Geometry: final body of the model. Coordinates: model frame, mm. A direction names the side the tool comes from. Coordinates: 2 decimals unless noted, no trailing zeros. Write each loop counter-clockwise with the first axis right and the second up, starting at its lowest first coordinate (ties: lowest second). Pieces come first, ordered by that corner, then holes. Notation, with made-up numbers: (-2.5, 22.5) - (48.5, 22.5) arc R10 cw to (48.5, 27.5) - close; hole circle Ø5 at (81, 62). An arc over 180 degrees is marked (long way). Answer as a JSON object with one key per item and string values. Group by question number.
Item 1: Set-up query: faces 1 (the flat face through (-9.5, 19, 3)), 2 (the flat face through (0, 5.65, 13)), 3 (the flat face through (7.825, 19, 16)). Return all of +Z, -Z, +X, -X, +Y, -Y with unobstructed straight access to the full face (end or side cutting, diameter ignored); none if empty.
Item 2: First-contact query: pin 1 Ø1.1 at (x, z) = (13, 3.5) entering from +Y; pin 2 Ø8 at (x, y) = (-20.5, 6.5) entering from +Z; pin 3 Ø3.5 at (x, y) = (20.5, 15.5) entering from -Z. Flat tips, straight axial feed; report the tip coordinate or a pass-through.
Item 3: Section C-C on z = -17.3. Return loops of the section in (x, y) (3 decimals), and give its area (3 significant figures).
Item 4: Line query: line 1 along X through (y, z) = (17.5, 3) (3 decimals); line 2 along Z through (x, y) = (2.5, 11); line 3 along X through (y, z) = (8.5, 0.5) (3 decimals). Output: solid intervals per line, ascending. Write a range as from..to.
Item 5: Section A-A on y = 10. Return loops of the section in (x, z) (3 decimals), and give its area (3 significant figures).
Item 6: Mould query, pull axis Z, two halves, no side actions, for faces 4 (the flat face through (0, 13.65, -17)), 5 (the flat face through (-0.1, 17.7, 18.85)), 6 (the flat face through (7.825, 13, -16)), 7 (the cylindrical face through (-0.06, 6.51, 9.75)). Classes: pulls with the +Z half, pulls with the -Z half, needs draft (parallel to the pull), parting line crosses it, or undercut.
Item 7: Section B-B on x = 0. Return loops of the section in (y, z), and give its area (3 significant figures).
```python
from build123d import *

# Parameters (mm, degrees)
SKETCH1_W             = 60
SKETCH1_H             = 18
BOSS_EXTRUDE1_DEPTH   = 26
SKETCH2_R             = 3.85
EYESHAFT_HOLES_DEPTH  = 15
EYESHAFT_FILLET_R     = 3
SKETCH5_W             = 5
SKETCH5_H             = 2.2
FRONT_LEG_HOLES_DEPTH = 13
SKETCH7_W             = 10.2
SKETCH7_H             = 3.3
BACK_LEGS_DEPTH       = 13
SKETCH18_W            = 15.65
SKETCH18_H            = 35.9
SERVO_BLOCK_DEPTH     = 26
SKETCH19_W            = 11.75
SKETCH19_H            = 32.2
SERVO_ARMS_DEPTH      = 9.35
SKETCH20_W            = 11.75
SKETCH20_H            = 23.9
CUT_EXTRUDE10_DEPTH   = 15
FILLET4_R             = 5
CHAMFER1_SIZE         = 1
SKETCH21_W            = 9
SKETCH21_H            = 4
CUT_EXTRUDE11_DEPTH   = 15
FILLET5_R             = 3
SKETCH22_R            = 0.75
CUT_EXTRUDE12_DEPTH   = 3
FILLET6_R             = 5
SKETCH23_W            = 15.65
SKETCH23_H            = 10
BOSS_EXTRUDE3_DEPTH   = 4
DOVE_TAIL_DEPTH       = 8
FILLET8_R             = 3.8
FILLET9_R             = 2


with BuildPart() as part:
    # Sketch1 → Boss-Extrude1 (new body)
    with BuildSketch(Plane(origin=(0, 0, 0), x_dir=(1, 0, 0), z_dir=(0, 1, 0))):
        Rectangle(SKETCH1_W, SKETCH1_H)
    extrude(amount=BOSS_EXTRUDE1_DEPTH)

    # Sketch2 → Eyeshaft holes (cut)
    with BuildSketch(Plane(origin=(0, 26, 0), x_dir=(1, 0, 0), z_dir=(0, 1, 0))):
        with Locations(Location((-22, -3, 0), (0, 0, 270))):
            Circle(SKETCH2_R)
        with Locations(Location((22, -3, 0), (0, 0, 270))):
            Circle(SKETCH2_R)
    extrude(amount=-EYESHAFT_HOLES_DEPTH, mode=Mode.SUBTRACT)

    # Eyeshaft Fillet
    eyeshaft_fillet_edges = [part.edges().sort_by_distance(p)[0] for p in [
        (-22, 11, -0.85),
        (22, 11, -0.85),
    ]]
    fillet(eyeshaft_fillet_edges, radius=EYESHAFT_FILLET_R)

    # Sketch5 → Front leg holes (cut)
    with BuildSketch(Plane(origin=(0, 26, 0), x_dir=(1, 0, 0), z_dir=(0, 1, 0))):
        with Locations((-12, -3)):
            Rectangle(SKETCH5_W, SKETCH5_H)
        with Locations((12, -3)):
            Rectangle(SKETCH5_W, SKETCH5_H)
    extrude(amount=-FRONT_LEG_HOLES_DEPTH, mode=Mode.SUBTRACT)

    # Sketch7 → Back Legs (cut)
    with BuildSketch(Plane(origin=(0, 26, 0), x_dir=(1, 0, 0), z_dir=(0, 1, 0))):
        with Locations((-13.9, 5.4)):
            Rectangle(SKETCH7_W, SKETCH7_H)
        with Locations((13.9, 5.4)):
            Rectangle(SKETCH7_W, SKETCH7_H)
    extrude(amount=-BACK_LEGS_DEPTH, mode=Mode.SUBTRACT)

    # Sketch18 → Servo Block (add)
    with BuildSketch(Plane(origin=(0, 26, 0), x_dir=(1, 0, 0), z_dir=(0, 1, 0))):
        with Locations((0, 3.1)):
            Rectangle(SKETCH18_W, SKETCH18_H)
    extrude(amount=-SERVO_BLOCK_DEPTH)

    # Sketch19 → Servo Arms (cut)
    with BuildSketch(Plane(origin=(0, 26, 0), x_dir=(1, 0, 0), z_dir=(0, 1, 0))):
        with Locations((0, 3.1)):
            Rectangle(SKETCH19_W, SKETCH19_H)
    extrude(amount=-SERVO_ARMS_DEPTH, mode=Mode.SUBTRACT)

    # Sketch20 → Cut-Extrude10 (cut)
    with BuildSketch(Plane(origin=(0, 16.65, 0), x_dir=(1, 0, 0), z_dir=(0, 1, 0))):
        with Locations((0, 3.1)):
            Rectangle(SKETCH20_W, SKETCH20_H)
    extrude(amount=-CUT_EXTRUDE10_DEPTH, mode=Mode.SUBTRACT)

    # Fillet4
    fillet4_edges = [part.edges().sort_by_distance(p)[0] for p in [
        (30, 13, 9),
        (-30, 13, 9),
        (-30, 13, -9),
        (30, 13, -9),
    ]]
    fillet(fillet4_edges, radius=FILLET4_R)

    # Chamfer1
    chamfer1_edges = [part.edges().sort_by_distance(p)[0] for p in [
        (-22, 26, -0.85),
        (22, 26, -0.85),
        (-9.5, 26, 3),
        (-12, 26, 1.9),
        (-14.5, 26, 3),
        (-12, 26, 4.1),
        (14.5, 26, 3),
        (12, 26, 1.9),
        (9.5, 26, 3),
        (12, 26, 4.1),
        (-19, 26, -5.4),
        (-13.9, 26, -3.75),
        (-8.8, 26, -5.4),
        (-13.9, 26, -7.05),
        (8.8, 26, -5.4),
        (13.9, 26, -3.75),
        (19, 26, -5.4),
        (13.9, 26, -7.05),
    ]]
    chamfer(chamfer1_edges, length=CHAMFER1_SIZE)

    # Sketch21 → Cut-Extrude11 (cut)
    with BuildSketch(Plane(origin=(0, 0, 8.85), x_dir=(-1, 0, 0), z_dir=(0, 0, -1))):
        with Locations((0, 3.65)):
            Rectangle(SKETCH21_W, SKETCH21_H)
    extrude(amount=-CUT_EXTRUDE11_DEPTH, mode=Mode.SUBTRACT)

    # Fillet5
    fillet5_edges = [part.edges().sort_by_distance(p)[0] for p in [
        (0, 5.65, 8.85),
    ]]
    fillet(fillet5_edges, radius=FILLET5_R)

    # Sketch22 → Cut-Extrude12 (cut)
    with BuildSketch(Plane(origin=(0, 16.65, 0), x_dir=(1, 0, 0), z_dir=(0, 1, 0))):
        with Locations(Location((0, 17.3, 0), (0, 0, 270))):
            Circle(SKETCH22_R)
        with Locations(Location((0, -11.1, 0), (0, 0, 270))):
            Circle(SKETCH22_R)
    extrude(amount=-CUT_EXTRUDE12_DEPTH, mode=Mode.SUBTRACT)

    # Fillet6
    fillet6_edges = [part.edges().sort_by_distance(p)[0] for p in [
        (-7.825, 13, -9),
        (-7.825, 13, 9),
        (7.825, 13, -9),
        (7.825, 13, 9),
    ]]
    fillet(fillet6_edges, radius=FILLET6_R)

    # Sketch23 → Boss-Extrude3 (add)
    with BuildSketch(Plane.XY.offset(14.85)):
        with Locations((0, 21)):
            Rectangle(SKETCH23_W, SKETCH23_H)
    extrude(amount=BOSS_EXTRUDE3_DEPTH)

    # Sketch24 → Dove tail (cut)
    with BuildSketch(Plane(origin=(0, 26, 0), x_dir=(1, 0, 0), z_dir=(0, 1, 0))):
        Polygon((6, -14.720854239), (-6, -14.720854239), (-3, -18.85), (3, -18.85), align=None)
    extrude(amount=-DOVE_TAIL_DEPTH, mode=Mode.SUBTRACT)

    # Fillet8
    fillet8_edges = [part.edges().sort_by_distance(p)[0] for p in [
        (0, 16, 14.85),
    ]]
    fillet(fillet8_edges, radius=FILLET8_R)

    # Fillet9
    fillet9_edges = [part.edges().sort_by_distance(p)[0] for p in [
        (7.825, 13, -21.05),
        (-7.825, 13, -21.05),
    ]]
    fillet(fillet9_edges, radius=FILLET9_R)


solid = part.part
```
Checks:
{
 "1": {"face 1": "+Y", "face 2": "+Z", "face 3": "+Z, +X, +Y, -Y"},
 "2": {"pin 1": "y = 13", "pin 2": "z = 9", "pin 3": "z = -9"},
 "3": {"outline": "(-7.825, 0) - (7.825, 0) - (7.825, 26) - (5.875, 26) - (5.875, 16.65) - (0.75, 16.65) - (0.75, 13.65) - (-0.75, 13.65) - (-0.75, 16.65) - (-5.875, 16.65) - (-5.875, 26) - (-7.825, 26) - close", "area": "293 mm^2"},
 "4": {"line 1": "-30..-25.85, -18.15..-14.5, -9.5..-5.875, 5.875..9.5, 14.5..18.15, 25.85..30", "line 2": "-21.05..-15.05, 8.85..14.85", "line 3": "-30..-5.875, 5.875..30"},
 "5": {"outline": "(-30, -4) arc R5 ccw to (-25, -9) - (-12.825, -9) arc R5 cw to (-7.825, -14) - (-7.825, -19.05) arc R2 ccw to (-5.825, -21.05) - (5.825, -21.05) arc R2 ccw to (7.825, -19.05) - (7.825, -14) arc R5 cw to (12.825, -9) - (25, -9) arc R5 ccw to (30, -4) - (30, 4) arc R5 ccw to (25, 9) - (12.825, 9) arc R5 cw to (7.825, 14) - (7.825, 14.85) - (-7.825, 14.85) - (-7.825, 14) arc R5 cw to (-12.825, 9) - (-25, 9) arc R5 ccw to (-30, 4) - close; hole (-5.875, -15.05) - (5.875, -15.05) - (5.875, 8.85) - (-5.875, 8.85) - close", "area": "1,080 mm^2"},
 "6": {"face 4": "undercut", "face 5": "pulls with the +Z half", "face 6": "needs draft", "face 7": "undercut"},
 "7": {"outline": "(0, -21.05) - (26, -21.05) - (26, -19.2) - (16.65, -19.2) - (16.65, -18.05) - (13.65, -18.05) - (13.65, -16.55) - (16.65, -16.55) - (16.65, -15.05) - (1.65, -15.05) - (1.65, 14.85) - (0, 14.85) - close; (5.65, 11.85) arc R3 ccw to (8.65, 8.85) - (16.65, 8.85) - (16.65, 10.35) - (13.65, 10.35) - (13.65, 11.85) - (16.65, 11.85) - (16.65, 13) - (26, 13) - (26, 14.72) - (18, 14.72) - (18, 18.85) - (16, 18.85) - (16, 18.65) arc R3.8 cw to (12.2, 14.85) - (5.65, 14.85) - close", "area": "249 mm^2"}
}
